Study the drawing (mm; zero at the part's minimum x, y, z) and answer. A direction names the side the tool comes from. Round coordinates to 2 decimals unless told otherwise and drop trailing zeros. Loops run counter-clockwise (first coordinate to the right, second up) from the corner with the lowest first, then second, coordinate; pieces in that order, holes last. Notation, with made-up numbers: (48, -38) - (74, -38) arc R14 ccw to (74, -23) - close; hole circle Ø4 at (-20.5, 65). An arc over 180 degrees is marked (long way). Use CSV: the item, a comma, the result in double quotes. Start each with the question number.
1. Determine the mould class of the marked faces 1, 2 and 3 for opening direction X: +X half, -X half, draft (parallel to the pull), parting line (faces both ways), or undercut.
2. Consider line 1 along Z through (x, y) = (2.1, 1.9); line 2 along Z through (x, y) = (2.1, 0.8); line 3 along X through (y, z) = (2.55, 8.5). Determine where each line is inside the solid, lowest interval first.
3. Given pin 1 Ø3 at (x, z) = (2, 5.5) entering from -Y; pin 2 Ø0.8 at (y, z) = (3, 11.5) entering from -X, each flat-ended and moving along its own axis, determine where each tip first touches the part or whether it passes through.
4. Find section A-A (y = 2.5). Give the vertices of the cut face in (x, z), and give its area (3 significant figures).
5. Find section D-D (x = 4.3). Give the vertices of the cut face in (y, z) (1 decimal), and give its area (3 significant figures).
6. Find section B-B (x = 2.2). Give the vertices of the cut face in (y, z), and give its area (3 significant figures).
7. Find section C-C (z = 9). Give the vertices of the cut face in (x, y).
8. A tool of negligible diameter and unlimited length cuts with its end or side. For the marked faces 4, 5 and 6, from which of +Z, -Z, +X, -X, +Y, -Y can it reach the whole face along a straight path? Write none if from no direction.
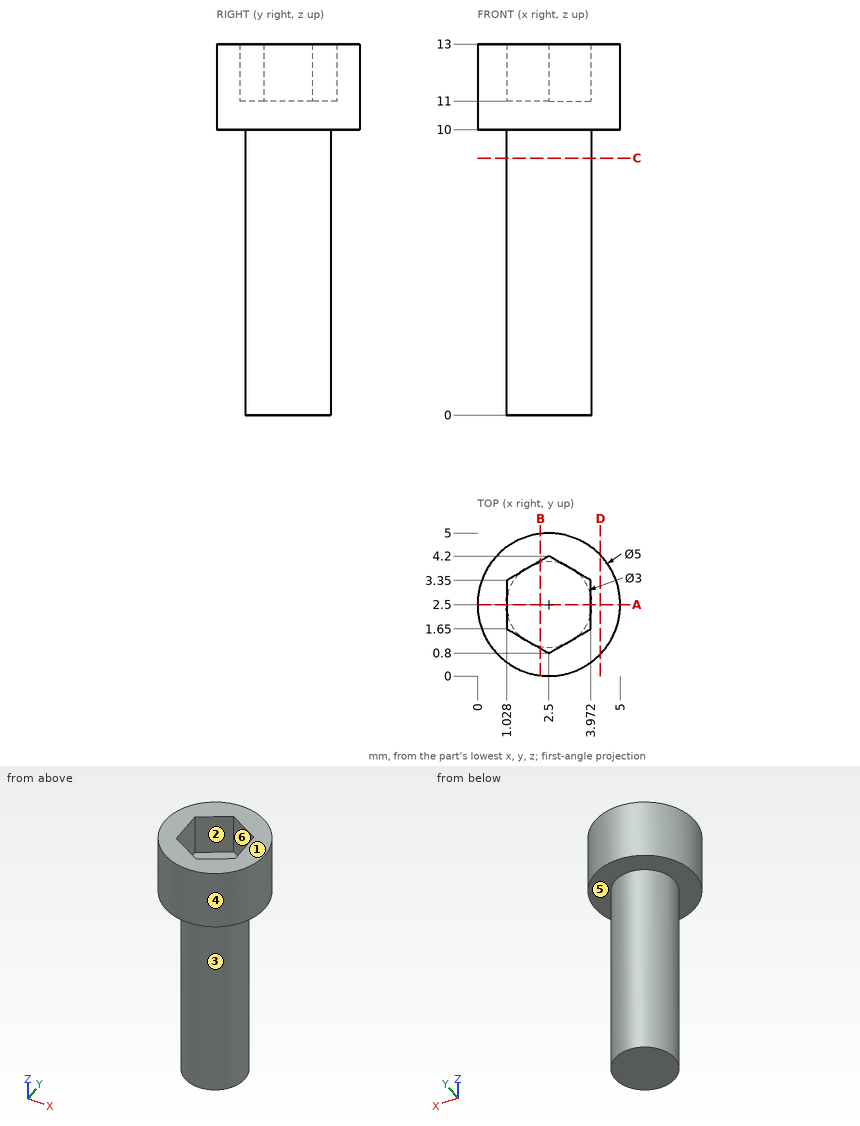
Filled sheet:
1,face 1,"draft"
1,face 2,"undercut"
1,face 3,"parting line"
2,line 1,"z = 0 to 11"
2,line 2,"z = 10 to 13"
2,line 3,"x = 1 to 4"
3,pin 1,"stops at y = 1"
3,pin 2,"stops at x = 0"
4,outline,"(0, 10) - (1, 10) - (1, 0) - (4, 0) - (4, 10) - (5, 10) - (5, 13) - (3.97, 13) - (3.97, 11) - (1.03, 11) - (1.03, 13) - (0, 13) - close"
4,area,"39.1 mm²"
5,outline,"(0.8, 10) - (4.2, 10) - (4.2, 13) - (0.8, 13) - close"
5,area,"10.4 mm²"
6,outline,"(0.02, 10) - (1.03, 10) - (1.03, 0) - (3.97, 0) - (3.97, 10) - (4.98, 10) - (4.98, 13) - (4.03, 13) - (4.03, 11) - (0.97, 11) - (0.97, 13) - (0.02, 13) - close"
6,area,"38.2 mm²"
7,outline,"circle Ø3 at (2.5, 2.5)"
8,face 4,"+Z, -Z"
8,face 5,"-Z"
8,face 6,"+Z"
